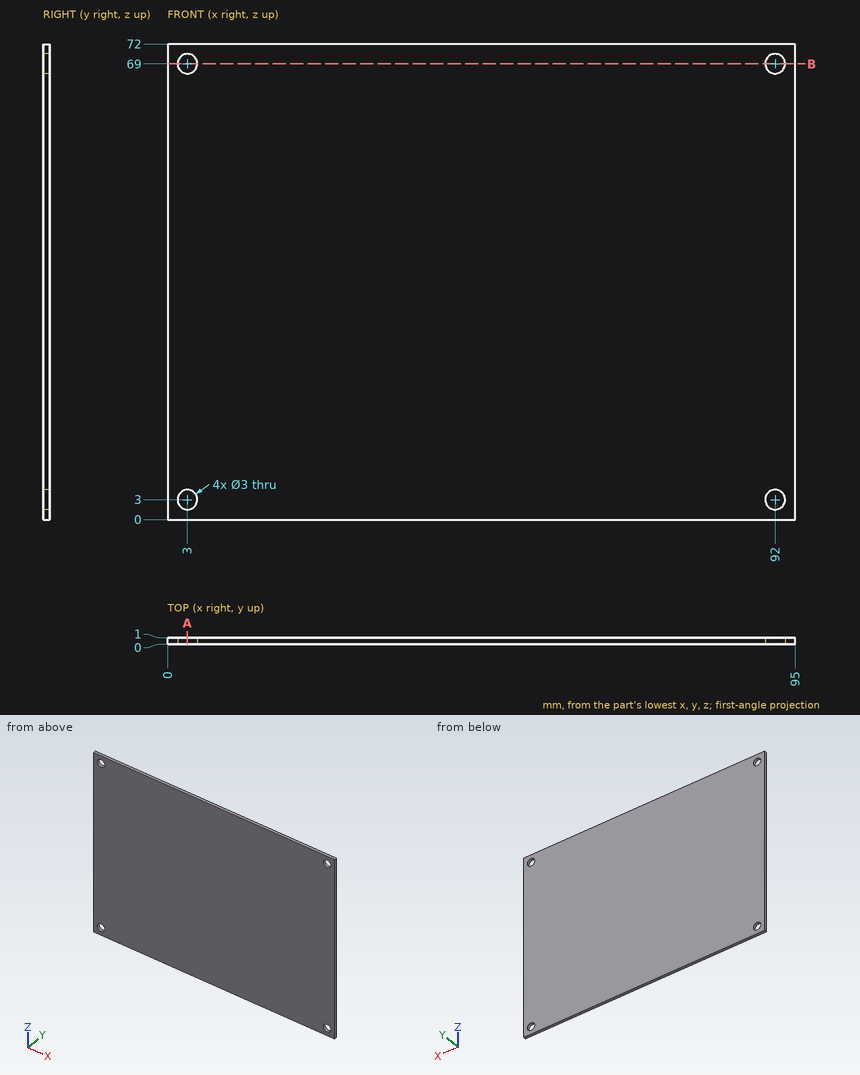
Can you work these out from the drawing? Everything is in mm from the part's minimum corner. Give positions to 0.01 mm unless a question says otherwise; leave off trailing zeros. Write each loop counter-clockwise with the first axis right and the second up, starting at its lowest first coordinate (ties: lowest second). Pieces come first, ordered by that corner, then holes. Notation, with made-up numbers: (52, 51.25) -> (94, 51.25) arc R24 ccw to (94, 76.25) -> close; hole circle Ø6 at (58, 53.5). An arc over 180 degrees is marked (long way). Write each question's results on one line, items separated by ' | '. Start each with the question number.
Q1. Suppose I cut it at A-A, the plane x = 3. List the corners of the cut face in (y, z) for me.
Q2. I need wall thicknesses on probe 1 along Z at (x, y) = (3, 0.65); probe 2 along X at (y, z) = (0.55, 69). Which ranges of each line are inside material? Lowest first, please.
Q3. Suppose I cut it at B-B, the plane z = 69. List the corners of the cut face in (x, y) for me.
Q4. I'm going to push a flat-ended pin straight in: pin 1 Ø1.5 at (x, z) = (41.5, 34.5) entering from -Y. Where does the tip first touch, or does it pass through?
Outcome:
1) outline: (0, 0) -> (1, 0) -> (1, 1.5) -> (0, 1.5) -> close; (0, 4.5) -> (1, 4.5) -> (1, 67.5) -> (0, 67.5) -> close; (0, 70.5) -> (1, 70.5) -> (1, 72) -> (0, 72) -> close
2) probe 1: 0 to 1.5, 4.5 to 67.5, 70.5 to 72 | probe 2: 0 to 1.5, 4.5 to 90.5, 93.5 to 95
3) outline: (0, 0) -> (1.5, 0) -> (1.5, 1) -> (0, 1) -> close; (4.5, 0) -> (90.5, 0) -> (90.5, 1) -> (4.5, 1) -> close; (93.5, 0) -> (95, 0) -> (95, 1) -> (93.5, 1) -> close
4) pin 1: y = 0
